The listing builds one solid part. Answer for the finished solid, in the listing's coordinates (mm). A direction names the side the tool comes from. Coordinates: 2 decimals unless noted, no trailing zeros. Loops run counter-clockwise (first coordinate to the right, second up) from the corner with the lowest first, then second, coordinate; pieces in that order, holes last. Notation, with made-up numbers: (-5.5, 62.5) - (25.5, 62.5) arc R25 cw to (25.5, 87.5) - close; hole circle Ø6 at (-10, -3.5). An arc over 180 degrees is marked (long way). Return JSON: item names as keys, results as strings. Group by question number.
1. Which of the six approach directions +Z, -Z, +X, -X, +Y, -Y give full straight-line access (tool end or side, diameter ignored) to faces 4 (the face through (-23.94, 20.12, 5.44)), 5 (the face through (25, -17.4, 9))?
2. Section D-D (x = 11.5) is taken. Write down the section's boundary in (y, z), and give its area (3 significant figures).
3. The mould has two halves that part along X. Classify faces 1 (the face through (-27.86, 0, 1)), 2 (the face through (0, 0, 3)), 3 (the face through (0, 0, 0)): pulls with the +X half, pulls with the -X half, needs draft (parallel to the pull), parting line crosses it, or undercut.
4. Find the intervals of material crossed by line 1 along Y through (x, z) = (-22.86, 6.25); line 2 along X through (y, z) = (17, 7.5); line 3 along X through (y, z) = (-14.5, 2.25), in increasing order.
5. Section C-C (y = -13.5) is taken. Write down the section's boundary in (x, z), and give its area (3 significant figures).
6. Section B-B (x = 24) is taken. Write down the section's boundary in (y, z), and give its area (3 significant figures).
7. This flat-tipped pin is pushed along its axis until it touches: P1, Ø3, axis at x = -22.86, y = -15.24, coming from the +Z side. Where does it stop, or does it pass through?
8. Section A-A (z = 6) is taken. Write down the section's boundary in (x, y).
Autodesk Fusion 360 part; units mm, degrees
sketch "Sketch1" plane through (0, 0, 0) normal (0, 0, 1) x (1, 0, 0)
  line L0 (22.86, -15.24) -> (-22.86, -15.24) construction
  line L1 (-22.86, -15.24) -> (-22.86, 15.24) construction
  line L2 (-22.86, 15.24) -> (22.86, 15.24) construction
  line L3 (22.86, 15.24) -> (22.86, -15.24) construction
  line L4 (22.86, -15.24) -> (-22.86, 15.24) construction
  line L5 (-22.86, -15.24) -> (22.86, 15.24) construction
  circle A0 centre (22.86, 15.24) radius 5
  circle A1 centre (22.86, -15.24) radius 5
  circle A2 centre (-22.86, -15.24) radius 5
  circle A3 centre (-22.86, 15.24) radius 5
  line L6 (-22.86, 20.24) -> (22.86, 20.24)
  line L7 (-27.86, 15.24) -> (-27.86, -15.24)
  line L8 (27.86, 15.24) -> (27.86, -15.24)
  line L9 (-22.86, -20.24) -> (22.86, -20.24)
  circle A4 centre (22.86, 15.24) radius 2.7
  circle A5 centre (-22.86, 15.24) radius 2.7
  circle A6 centre (-22.86, -15.24) radius 2.7
  circle A7 centre (22.86, -15.24) radius 2.7
  dimension "d1" = 45.72
  dimension "d2" = 30.48
  dimension "d3" = 10
  dimension "d4" = 10
  dimension "d5" = 10
  dimension "d6" = 10
  dimension "d12" = 5.4
  dimension "d13" = 5.4
  dimension "d14" = 5.4
  dimension "d15" = 5.4
extrude "Extrude1" add sketch "Sketch1" along normal blind 3 contours A0 | A0 A1 A2 A3 L6 L7 L8 L9 | A1 | A3 | A2 | A4 | A5 | A6 | A7
extrude "Extrude2" add sketch "Sketch1" along normal blind 6 from surface at 3 contours A0 | A1 | A3 | A2 | A4 | A5 | A6 | A7
extrude "Extrude3" cut sketch "Sketch1" against normal blind 7 from surface at 9 contours A4 | A5 | A6 | A7
equation "d4 = d3"
equation "d5 = d3"
equation "d6 = d3"
equation "d13 = d12"
equation "d14 = d12"
equation "d15 = d12"
The answers:
{
 "1": {"face 4": "+Z", "face 5": "+Z, +X, -X, +Y, -Y"},
 "2": {"outline": "(-20.24, 0) - (20.24, 0) - (20.24, 3) - (-20.24, 3) - close", "area": "121 mm2"},
 "3": {"face 1": "pulls with the -X half", "face 2": "undercut", "face 3": "needs draft"},
 "4": {"line 1": "y = -20.24 to -17.94, -12.54 to -10.24, 10.24 to 12.54, 17.94 to 20.24", "line 2": "x = -27.54 to -24.91, -20.81 to -18.18, 18.18 to 20.81, 24.91 to 27.54", "line 3": "x = -27.86 to -25.46, -20.26 to 20.26, 25.46 to 27.86"},
 "5": {"outline": "(-27.86, 0) - (27.86, 0) - (27.86, 3) - (27.55, 3) - (27.55, 9) - (24.92, 9) - (24.92, 2) - (20.8, 2) - (20.8, 9) - (18.17, 9) - (18.17, 3) - (-18.17, 3) - (-18.17, 9) - (-20.8, 9) - (-20.8, 2) - (-24.92, 2) - (-24.92, 9) - (-27.55, 9) - (-27.55, 3) - (-27.86, 3) - close", "area": "222 mm2"},
 "6": {"outline": "(-20.11, 0) - (20.11, 0) - (20.11, 9) - (17.69, 9) - (17.69, 2) - (12.79, 2) - (12.79, 9) - (10.37, 9) - (10.37, 3) - (-10.37, 3) - (-10.37, 9) - (-12.79, 9) - (-12.79, 2) - (-17.69, 2) - (-17.69, 9) - (-20.11, 9) - close", "area": "169 mm2"},
 "7": {"P1": "stops at z = 2"},
 "8": {"outline": "circle Ø10 at (-22.86, -15.24); circle Ø10 at (-22.86, 15.24); circle Ø10 at (22.86, -15.24); circle Ø10 at (22.86, 15.24); hole circle Ø5.4 at (-22.86, -15.24); hole circle Ø5.4 at (-22.86, 15.24); hole circle Ø5.4 at (22.86, -15.24); hole circle Ø5.4 at (22.86, 15.24)"}
}
